```python
from build123d import *

# Parameters (mm, degrees)
BOSS_EXTRUDE1_DEPTH = 3.81
CUT_EXTRUDE1_REACH  = 87.779
SKETCH2_R           = 2.447521694
SKETCH2_R_2         = 2.514751493
SKETCH2_R_3         = 2.570723965
SKETCH2_R_4         = 2.649131916


with BuildPart() as part:
    # Sketch1 → Boss-Extrude1 (new body)
    with BuildSketch(Plane.XY):
        with BuildLine():
            Line((55.88, -54.61), (-55.88, -54.61))
            ThreePointArc((-55.88, -54.61), (-63.064204897, -51.634204897), (-66.04, -44.45))
            Line((-66.04, -44.45), (-66.04, 44.45))
            ThreePointArc((-66.04, 44.45), (-63.064204897, 51.634204897), (-55.88, 54.61))
            Line((-55.88, 54.61), (55.88, 54.61))
            ThreePointArc((55.88, 54.61), (63.064204897, 51.634204897), (66.04, 44.45))
            Line((66.04, 44.45), (66.04, -44.45))
            ThreePointArc((66.04, -44.45), (63.064204897, -51.634204897), (55.88, -54.61))
        make_face()
    extrude(amount=BOSS_EXTRUDE1_DEPTH)

    # Sketch2 → Cut-Extrude1 (cut, up to next)
    with BuildSketch(Plane.XY.offset(3.81), mode=Mode.PRIVATE) as cut_extrude1_sk1:
        with Locations((-55.936087501, 46.99)):
            Circle(SKETCH2_R)
    cut_extrude1_tool1 = extrude(cut_extrude1_sk1.sketch, amount=-CUT_EXTRUDE1_REACH, mode=Mode.PRIVATE) & part.part
    # Sketch2 → Cut-Extrude1 (cut, up to next)
    with BuildSketch(Plane.XY.offset(3.81), mode=Mode.PRIVATE) as cut_extrude1_sk2:
        with Locations((56.105983157, 46.99)):
            Circle(SKETCH2_R_2)
    cut_extrude1_tool2 = extrude(cut_extrude1_sk2.sketch, amount=-CUT_EXTRUDE1_REACH, mode=Mode.PRIVATE) & part.part
    # Sketch2 → Cut-Extrude1 (cut, up to next)
    with BuildSketch(Plane.XY.offset(3.81), mode=Mode.PRIVATE) as cut_extrude1_sk3:
        with Locations((56.105983157, -44.758153673)):
            Circle(SKETCH2_R_3)
    cut_extrude1_tool3 = extrude(cut_extrude1_sk3.sketch, amount=-CUT_EXTRUDE1_REACH, mode=Mode.PRIVATE) & part.part
    # Sketch2 → Cut-Extrude1 (cut, up to next)
    with BuildSketch(Plane.XY.offset(3.81), mode=Mode.PRIVATE) as cut_extrude1_sk4:
        with Locations((-56.244241173, -44.758153673)):
            Circle(SKETCH2_R_4)
    cut_extrude1_tool4 = extrude(cut_extrude1_sk4.sketch, amount=-CUT_EXTRUDE1_REACH, mode=Mode.PRIVATE) & part.part
    add(cut_extrude1_tool1.solids().sort_by_distance((-55.936088, 46.99, 3.81))[0], mode=Mode.SUBTRACT)
    add(cut_extrude1_tool2.solids().sort_by_distance((56.105983, 46.99, 3.81))[0], mode=Mode.SUBTRACT)
    add(cut_extrude1_tool3.solids().sort_by_distance((56.105983, -44.758154, 3.81))[0], mode=Mode.SUBTRACT)
    add(cut_extrude1_tool4.solids().sort_by_distance((-56.244241, -44.758154, 3.81))[0], mode=Mode.SUBTRACT)


solid = part.part
```
Here's how the part is built. I have some questions about the finished solid (model axes, mm). Coordinates: 2 decimals unless noted, no trailing zeros. Order: outer loops, then holes, each group sorted by start corner. A loop starts at its lowest first (then second) coordinate and runs counter-clockwise, first axis right, second up.
Item 1: I need wall thicknesses on probe 1 along Y at (x, z) = (56.5, 1.6); probe 2 along Y at (x, z) = (54, 1.9); probe 3 along X at (y, z) = (47.5, 1.7). Which ranges of each line are inside material? Lowest first, please.
Response values:
probe 1: y = -54.59 to -47.3, -42.22 to 44.51, 49.47 to 54.59
probe 2: y = -54.61 to -46.23, -43.28 to 45.62, 48.36 to 54.61
probe 3: x = -65.57 to -58.33, -53.54 to 53.64, 58.57 to 65.57
Item 2: If we section it at A-A, the plane y = 46.99: List the corners of the cut face in (x, z) for me, then the cut area to 3 significant figures.
Response values:
outline: (-65.72, 0) - (-58.38, 0) - (-58.38, 3.81) - (-65.72, 3.81) - close; (-53.49, 0) - (53.59, 0) - (53.59, 3.81) - (-53.49, 3.81) - close; (58.62, 0) - (65.72, 0) - (65.72, 3.81) - (58.62, 3.81) - close
area: 463 mm2
Item 3: Thinking about a two-plate mould opening in X: for faces 1 (the face through (63.1, -51.6, 1.9)), 2 (the face through (-66.04, -1, 2)), 3 (the face through (-1, 54.61, 2)), 4 (the face through (54.066, -46.322, 1.932)), which applies, pulls with the +X half, pulls with the -X half, needs draft (parallel to the pull), parting line crosses it, or undercut?
Response values:
face 1: pulls with the +X half
face 2: pulls with the -X half
face 3: needs draft
face 4: undercut
Item 4: I'm going to push a flat-ended pin straight in: pin 1 Ø3 at (x, y) = (56.11, 46.99) entering from +Z. Where does the tip first touch, or does it pass through?
Response values:
pin 1: passes through
